Could you check a few things on this model? Use its own coordinates, in mm. Face numbers are marked on the shaded views. A direction names the side the tool comes from. Coordinates: 2 decimals unless noted, no trailing zeros. Loops run counter-clockwise (first coordinate to the right, second up) from the corner with the lowest first, then second, coordinate; pieces in that order, holes last. Notation, with made-up numbers: (40.25, 36) - (85.25, 36) arc R19 cw to (85.25, 58) - close; hole circle Ø9 at (74.25, -21). An arc over 180 degrees is marked (long way). One line per item, written item: value. Start each with the question number.
(1) On a 3-axis mill with a long thin cutter (end or side, diameter ignored), from which of +Z, -Z, +X, -X, +Y, -Y can I reach the whole of each face in a straight line? I mean the marked faces 4, 5 and 6. Say none if no direction works.
(2) If I drill on line 1 along Y through (x, z) = (6.25, 11.25); line 2 along X through (y, z) = (-30, 9); line 3 along X through (y, z) = (-38, 3.25), over which ranges is the centre line in solid material (lowest first)? Write a range as from..to.
(3) If we section it at C-C on y = -46: Write out the boundary of the cut face in (x, z) (3 decimals), then the cut area to 3 significant figures.
(4) If we mould it in two halves opening along X, with no side actions, what happens to the marked faces 1, 2 and 3? For each: pulls with the +X half, pulls with the -X half, needs draft (parallel to the pull), parting line crosses it, or undercut.
(5) I'm going to push flat-ended pins straight in: P1, Ø12, axis at x = 2.5, y = -33.5, coming from the -Z side; P2, Ø1, axis at x = 3.5, z = 2, coming from the +Y side; P3, Ø3, axis at y = -8.5, z = 19.5, coming from the -X side; P4, Ø7, axis at x = -2.5, y = -35.5, coming from the +Z side (3 decimals). Where does each tip first touch, or does it pass through?
(6) If we section it at A-A on y = -37: Write out the boundary of the cut face in (x, z) (3 decimals).
(7) If we section it at B-B on y = -7.5: Write out the boundary of the cut face in (x, z) (3 decimals), then the cut area to 3 significant figures.
```python
from build123d import *

# Parameters (mm, degrees)
F1_W      = 36.2
F1_H      = 68.8
F2_W      = 12.866667
F2_H      = 68.8
F3_FACE_W = 36.2
F3_FACE_H = 68.8
F4_DEPTH  = 12
F5_W      = 13.8
F5_H      = 13.8
F6_DEPTH  = 31
F7_W      = 20
F7_H      = 34.4
F8_DEPTH  = 3.2


with BuildPart() as f3:
    # F1 (on offset) → F3 section 0
    with BuildSketch(Plane.XY.offset(36.125)):
        with Locations((0, -34.4)):
            Rectangle(F1_W, F1_H)
    # F2 (on Top) → F3 section 1
    with BuildSketch(Plane.XY):
        with Locations((-3.3e-05, -34.4)):
            Rectangle(F2_W, F2_H)
    loft()

    # F3_face (on face) → F4 (cut)
    with BuildSketch(Plane(origin=(0, -34.4, 36.125), x_dir=(1, 0, 0), z_dir=(0, 0, 1))):
        Rectangle(F3_FACE_W, F3_FACE_H)
    extrude(amount=-F4_DEPTH, mode=Mode.SUBTRACT)

    # F5 (on offset) → F6 (cut)
    with BuildSketch(Plane.XY.offset(36.125)):
        with Locations((0, -34.4)):
            Rectangle(F5_W, F5_H)
    extrude(amount=-F6_DEPTH, mode=Mode.SUBTRACT)

    # F7 (on Top) → F8 (cut)
    with BuildSketch(Plane.XY):
        with Locations((0, -34.4)):
            Rectangle(F7_W, F7_H)
    extrude(amount=F8_DEPTH, mode=Mode.SUBTRACT)


solid = f3.part
```
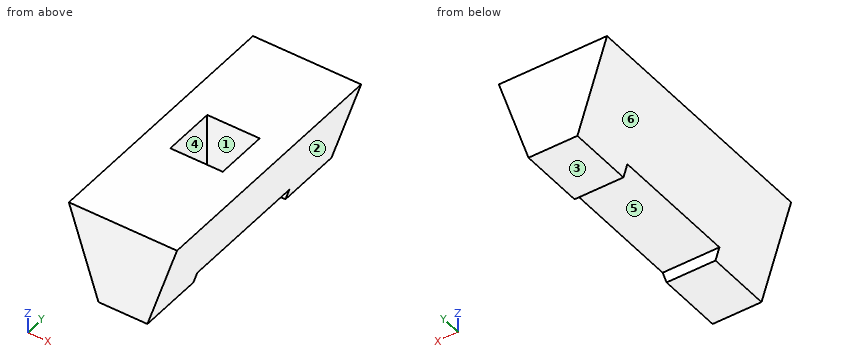
Values:
1. face 4: +Z
1. face 5: -Z, +X, -X
1. face 6: -Z, -X, +Y, -Y
2. line 1: y = -68.8..-41.3, -27.5..0
2. line 2: x = -9.34..-6.9, 6.9..9.34
2. line 3: x = -7.48..7.48
3. outline: (-14.225, 24.125) - (-7.467, 3.2) - (7.467, 3.2) - (14.225, 24.125) - close
3. area: 454 mm2
4. face 1: undercut
4. face 2: pulls with the +X half
4. face 3: needs draft
5. P1: stops at z = 3.2
5. P2: stops at y = 0
5. P3: stops at x = -13.22
5. P4: stops at z = 5.125
6. outline: (-14.225, 24.125) - (-7.467, 3.2) - (7.467, 3.2) - (14.225, 24.125) - (6.9, 24.125) - (6.9, 5.125) - (-6.9, 5.125) - (-6.9, 24.125) - close
7. outline: (-14.225, 24.125) - (-6.433, 0) - (6.433, 0) - (14.225, 24.125) - close
7. area: 498 mm2
